Work out the finished part from the listing and answer in its coordinate system (mm). A direction names the side the tool comes from. Give positions to 0.01 mm unless a question says otherwise; leave off trailing zeros. Write each loop counter-clockwise with the first axis right and the second up, starting at its lowest first coordinate (ties: lowest second). Pieces come first, ordered by that corner, then holes. Notation, with made-up numbers: (2, -9) - (7, -9) arc R8 cw to (7, -4) - close; hole circle Ø1 at (53, 40.25). An arc over 180 degrees is marked (long way). Write item = value, one per line.
Autodesk Inventor part; units mm, degrees
ref_plane "YZ Plane" through (0, 0, 0) normal (1, 0, 0) x (0, 1, 0)
ref_plane "XZ Plane" through (0, 0, 0) normal (0, 1, 0) x (-1, 0, 0)
ref_plane "XY Plane" through (0, 0, 0) normal (0, 0, 1) x (1, 0, 0)
sketch "Sketch29" plane through (0, 0, 0) normal (1, 0, 0) x (0, 1, 0)
  line L0 (0, 0) -> (1270, 0)
  line L1 (1270, 0) -> (1270, 508)
  line L2 (1270, 508) -> (0, 508)
  line L3 (0, 508) -> (0, 0)
  dimension "d230" = 508
  dimension "d231" = 1270
extrude "Plate26" add sketch "Sketch29" along normal blind 6.35
sketch "Sketch30" plane through (-0.2216, 1263.6539, 508) normal (0.0348995, 0.9993908, 0) x (-0.9993908, 0.0348995, 0)
  line L0 (0, -508) -> (0, 0)
  line L1 (0, 0) -> (-101.6, 0)
  line L2 (-101.6, 0) -> (-101.6, -508)
  line L3 (-101.6, -508) -> (0, -508)
edge flange "Flange23" height 101.6 angle 92 thickness 6.35 bend radius 6.35 thickness toward (0.0348995, 0.9993908, 0) relief tear relief width 6.35 relief depth 3.175 edges at (6.35, 1270, 254) wall of the first edge with corners at (-0.2216, 1263.6539, 0) (-0.2216, 1263.6539, 508) (101.3165, 1260.1081, 508) (101.3165, 1260.1081, 0)
bend "Bend23"
corner "Corner22"
equation "\"d230\" = LARGO"
equation "\"d231\" = ALTO"
equation "\"d237\" = LARGOF"
equation "\"d238\" = ANGULOF"
equation "\"BendRadius\" = Thickness"
equation "\"BendReliefWidth\" = Thickness"
equation "\"BendReliefDepth\" = 0.5 * Thickness"
equation "\"CornerReliefSize\" = 4 * Thickness"
equation "\"MinimumRemnant\" = 2 * Thickness"
equation "\"TransitionRadius\" = BendRadius"
equation "\"JacobiRadiusSize\" = BendRadius"
equation "\"GapSize\" = Thickness"
equation "\"LARGO\" = 508"
equation "\"ALTO\" = 1270"
equation "\"LARGOF\" = 101.6"
equation "\"ANGULOF\" = 92deg"
properties part number "BackWallTop" material "Carbon Steel - A36"
1. Given pin 1 (3 mm diameter, centred on x = 19.5, z = 79, fed in from +Y); pin 2 (3 mm diameter, centred on x = 44, z = 221, fed in from +Y); pin 3 (1.5 mm diameter, centred on x = 35, z = 438, fed in from -Y), each flat-ended and moving along its own axis, determine where each tip first touches the part or whether it passes through.
Solution:
pin_1 = 1269.37
pin_2 = 1268.52
pin_3 = 1262.4
2. Find section B-B, the plane y = 1186.5. Give the vertices of the cut face in (x, z), then the cut area to 3 significant figures.
Solution:
outline = (0, 0) - (6.35, 0) - (6.35, 508) - (0, 508) - close
area = 3,230 mm^2
3. Straight lines are drawn through the part: line 1 (Y direction, x = 95, z = 151); line 2 (X direction, y = 540.5, z = 301); line 3 (Y direction, x = 85.5, z = 58). For each, find the intervals that lie inside material, in ascending order.
Solution:
line_1 = 1260.33 to 1266.68
line_2 = 0 to 6.35
line_3 = 1260.66 to 1267.01
4. A tool of negligible diameter and unlimited length cuts with its end or side. For faces 1 (the flat face through (6.35, 620, 258)), 2 (the flat face through (6, 638, 508)), from which of +Z, -Z, +X, -X, +Y, -Y can it reach the whole face along a straight path? Write none if from no direction.
Solution:
face_1 = +Z, -Z, +X, -Y
face_2 = +Z, +X, -X, +Y, -Y
5. Find section A-A, the plane z = 44.5. Give the vertices of the cut face in (x, y).
Solution:
outline = (0, 0) - (6.35, 0) - (6.35, 1256.85) arc R6.35 cw to (12.92, 1263.19) - (101.32, 1260.11) - (101.54, 1266.45) - (13.14, 1269.54) arc R12.7 ccw to (0, 1256.85) - close
6. Find section C-C, the plane x = 62.5. Give the vertices of the cut face in (y, z).
Solution:
outline = (1261.46, 0) - (1267.82, 0) - (1267.82, 508) - (1261.46, 508) - close
